Input: part model. Units: mm. Frame: model coordinates. A direction names the side the tool comes from. Give positions to 0.01 mm unless a question says otherwise; leave off trailing zeros. Loops run counter-clockwise (first coordinate to the right, second up) from the corner with the lowest first, then second, coordinate; pieces in that order, holes last.
from build123d import *

# Parameters (mm, degrees)
BOSS_EXTRUDE1_DEPTH      = 5
M2_CLEARANCE_HOLE1_D     = 2.4
M2_CLEARANCE_HOLE1_DEPTH = 12
M2_CLEARANCE_HOLE1_TIP   = 0.721032743
SKETCH6_R                = 1.215
CUT_EXTRUDE1_DEPTH       = 10


with BuildPart() as part:
    # Sketch1 → Boss-Extrude1 (new body)
    with BuildSketch(Plane(origin=(0, 0, 0), x_dir=(1, 0, 0), z_dir=(0, 1, 0))):
        with BuildLine():
            Line((4.958856711, -28.278101888), (4.958856711, -16.278101888))
            Line((4.958856711, -16.278101888), (4.958856711, -13.505087823))
            Line((4.958856711, -13.505087823), (-12.812745649, -13.505087823))
            Line((-12.812745649, -13.505087823), (-12.812745649, -16.278101888))
            Line((-12.812745649, -16.278101888), (-12.812745649, -23.605635188))
            Line((-12.812745649, -23.605635188), (-4.368523326, -23.605635188))
            Line((-4.368523326, -23.605635188), (-4.368523326, -28.278101888))
            ThreePointArc((-4.368523326, -28.278101888), (0.295166692, -32.941791906), (4.958856711, -28.278101888))
        make_face()
    extrude(amount=BOSS_EXTRUDE1_DEPTH)

    # M2 Clearance Hole1
    with Locations(Plane(origin=(0, 5, 0), x_dir=(1, 0, 0), z_dir=(0, 1, 0))):
        with Locations((-0.041143289, -19.005087823), (-7.812745649, -19.005087823)):
            Hole(M2_CLEARANCE_HOLE1_D / 2, depth=M2_CLEARANCE_HOLE1_DEPTH)
            with Locations((0, 0, -(M2_CLEARANCE_HOLE1_DEPTH + M2_CLEARANCE_HOLE1_TIP / 2))):  # 118° drill point
                Cone(0, M2_CLEARANCE_HOLE1_D / 2, M2_CLEARANCE_HOLE1_TIP, mode=Mode.SUBTRACT)

    # Sketch6 → Cut-Extrude1 (cut)
    with BuildSketch(Plane(origin=(0, 5, 0), x_dir=(1, 0, 0), z_dir=(0, 1, 0))):
        with Locations((0.295166692, -28.278101888)):
            Circle(SKETCH6_R)
    extrude(amount=-CUT_EXTRUDE1_DEPTH, mode=Mode.SUBTRACT)


solid = part.part
(1) Mould query, pull axis X, two halves, no side actions, for faces 1 (the flat face through (-4.369, 2, 26)), 2 (the cylindrical face through (0.032, 2.535, 29.464)), 3 (the flat face through (-2, 0, 21)). Classes: +X half, -X half, draft (parallel to the pull), parting line (faces both ways), or undercut.
Values follow:
face 1: -X half
face 2: undercut
face 3: draft
(2) Cut plane A-A (x = 0.25). Return the cut outline in (y, z), and give its area (3 significant figures).
Values follow:
outline: (0, 13.51) - (5, 13.51) - (5, 17.84) - (0, 17.84) - close; (0, 20.17) - (5, 20.17) - (5, 27.06) - (0, 27.06) - close; (0, 29.49) - (5, 29.49) - (5, 32.94) - (0, 32.94) - close
area: 73.4 mm2
(3) Ray query, probe 1 along X at (y, z) = (3.7, 18); probe 2 along X at (y, z) = (2.65, 18.75); probe 3 along Z at (x, y) = (0.75, 4.25). Return the intervals inside material, ascending.
Values follow:
probe 1: x = -12.81 to -8.47, -7.16 to -0.7, 0.61 to 4.96
probe 2: x = -12.81 to -8.99, -6.64 to -1.21, 1.13 to 4.96
probe 3: z = 13.51 to 18.1, 19.91 to 27.15, 29.4 to 32.92
(4) Cut plane C-C (y = 1). Return the cut outline in (x, z) (3 decimals).
Values follow:
outline: (-12.813, 13.505) - (4.959, 13.505) - (4.959, 28.278) arc R4.664 ccw to (-4.369, 28.278) - (-4.369, 23.606) - (-12.813, 23.606) - close; hole circle Ø2.4 at (-7.813, 19.005); hole circle Ø2.4 at (-0.041, 19.005); hole circle Ø2.43 at (0.295, 28.278)
(5) Pin query (flat end, axial travel): pin 1 Ø1.5 at (x, z) = (0.3, 28.28) entering from -Y; pin 2 Ø1.5 at (x, y) = (-9, 2) entering from +Z. Return the tip coordinate at first contact, or that it passes through.
Values follow:
pin 1: passes through
pin 2: stops at z = 23.61
(6) Cut plane D-D (x = -10). Return the cut outline in (y, z), and give its area (3 significant figures).
Values follow:
outline: (0, 13.51) - (5, 13.51) - (5, 23.61) - (0, 23.61) - close
area: 50.5 mm2
(7) Cut plane B-B (z = 27.75). Return the cut outline in (x, y).
Values follow:
outline: (-4.37, 0) - (-0.8, 0) - (-0.8, 5) - (-4.37, 5) - close; (1.39, 0) - (4.96, 0) - (4.96, 5) - (1.39, 5) - close
(8) Reachability of faces 4 (the flat face through (-2, 5, 21)), 5 (the flat face through (-9, 2, 23.606)) from +Z, -Z, +X, -X, +Y, -Y: full face, straight path, thin tool, end or side. Return the list, or none.
Values follow:
face 4: +Z, -Z, +X, -X, +Y
face 5: +Z, -X, +Y, -Y
